Can you work these out from the model? Positions are in its coordinate system, mm. Face numbers are marked on the shaded views. A direction names the side the tool comes from. Coordinates: 2 decimals unless noted, no trailing zeros. Loops run counter-clockwise (first coordinate to the right, second up) from the corner with the lowest first, then second, coordinate; pieces in that order, holes last. Notation, with made-up numbers: M -13,8 L -5,8 A25 cw -5,27 Z; hole C 0,-33 d9. An arc over 180 degrees is marked long. Answer as a JSON object with one key per item and string values. Group by question number.
Item 1: I'm going to push flat-ended pins straight in: pin 1 Ø10 at (x, y) = (131, -83) entering from -Z; pin 2 Ø1.5 at (y, z) = (841, 21.5) entering from -X. Where does each tip first touch, or does it pass through?
Item 2: Suppose I cut it at A-A (x = 0). Write out the boundary of the cut face in (y, z), then the cut area to 3 significant figures.
Item 3: If I drill on line 1 (Y direction, x = 0, z = 54); line 2 (X direction, y = 892, z = 84); line 3 (Z direction, x = 321, y = -43.5), over which ranges is the centre line in solid material (lowest first)?
Item 4: Suppose I cut it at C-C (x = 369.5). Write out the boundary of the cut face in (y, z), then the cut area to 3 significant figures.
Item 5: Suppose I cut it at B-B (y = 0). Write out the boundary of the cut face in (x, z), then the cut area to 3 significant figures.
Item 6: Suppose I cut it at D-D (z = -72). Write out the boundary of the cut face in (x, y).
Item 7: Which directions (+Z, -Z, +X, -X, +Y, -Y) give clear straight access to the entire face, cutting with the end or side of a thin tool? Please do the marked faces 1, 2, 3 and 4.
```python
from build123d import *

# Parameters (mm, degrees)
SKETCH_1_W          = 1000
SKETCH_1_H          = 500
EXTRUDE_1_DEPTH     = 100
SKETCH_2_W          = 200
SKETCH_2_H          = 500
EXTRUDE_2_DEPTH     = 800
SKETCH_3_R          = 50
CUT_EXTRUDE_1_DEPTH = 1190.537725337


with BuildPart() as part:
    # 草图1 → 凸台-拉伸1 (new body)
    with BuildSketch(Plane.XY):
        Rectangle(SKETCH_1_W, SKETCH_1_H)
    extrude(amount=EXTRUDE_1_DEPTH)

    # 草图2 → 凸台-拉伸2 (add)
    with BuildSketch(Plane(origin=(0, 250, 0), x_dir=(1, 0, 0), z_dir=(0, 1, 0))):
        with Locations((400, 0)):
            Rectangle(SKETCH_2_W, SKETCH_2_H)
    extrude(amount=EXTRUDE_2_DEPTH)

    # 草图3 → 切除-拉伸1 (cut, through all)
    with BuildSketch(Plane.XY):
        with Locations(Location((0, 0, 0), (0, 0, 180))):
            Circle(SKETCH_3_R)
    extrude(amount=CUT_EXTRUDE_1_DEPTH, mode=Mode.SUBTRACT)


solid = part.part
```
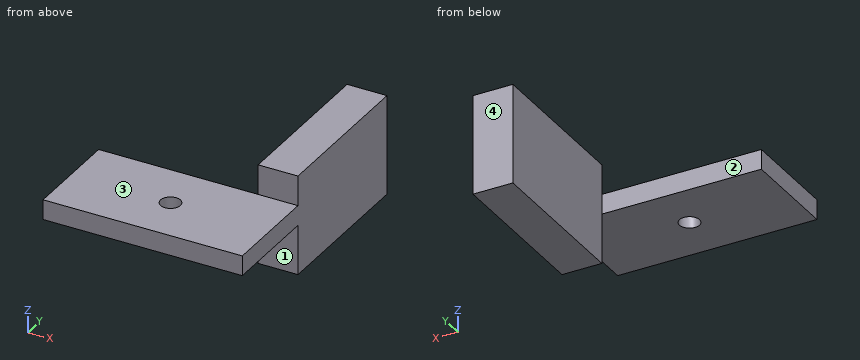
From the geometry:
{
 "1": {"pin 1": "z = 0", "pin 2": "x = 300"},
 "2": {"outline": "M -250,0 L -50,0 L -50,100 L -250,100 Z; M 50,0 L 250,0 L 250,100 L 50,100 Z", "area": "40,000 mm2"},
 "3": {"line 1": "-250 to -50, 50 to 250", "line 2": "300 to 500", "line 3": "0 to 100"},
 "4": {"outline": "M -250,0 L 250,0 L 250,-250 L 1050,-250 L 1050,250 L 250,250 L 250,100 L -250,100 Z", "area": "450,000 mm2"},
 "5": {"outline": "M -500,0 L -50,0 L -50,100 L -500,100 Z; M 50,0 L 500,0 L 500,100 L 50,100 Z", "area": "90,000 mm2"},
 "6": {"outline": "M 300,250 L 500,250 L 500,1050 L 300,1050 Z"},
 "7": {"face 1": "-Z, +X, -X, -Y", "face 2": "+Z, -Z, -X, +Y", "face 3": "+Z, +X, -X, -Y", "face 4": "+Z, -Z, +X, -X, +Y"}
}
